Model file for the job. Use its own axes, mm. Face numbers are marked on the shaded views. A direction names the side the tool comes from. Give positions to 0.01 mm unless a question says otherwise; leave off trailing zeros. Write each loop counter-clockwise with the first axis right and the second up, starting at its lowest first coordinate (ties: lowest second). Pieces come first, ordered by that corner, then holes. Notation, with made-up numbers: M -18,85.5 L 34,85.5 A24 ccw 34,97.5 Z; hole C -27.75,71 d3. An arc over 180 degrees is marked long. Answer as a JSON object with one key per item and string values. Group by question number.
```python
from build123d import *

# Parameters (mm, degrees)
SKETCH1_R           = 7.9375
BOSS_EXTRUDE1_DEPTH = 1.524


with BuildPart() as part:
    # Sketch1 → Boss-Extrude1 (new body)
    with BuildSketch(Plane.XY):
        with Locations(Location((107.492585866, -0.762, 0), (0, 0, 180))):
            Circle(SKETCH1_R)
        Polygon((110.207675722, 0), (110.207675722, -1.524), (108.925853356, -1.524), (108.869130969, -1.622246056), (109.510042152, -2.732336789), (108.190219437, -3.494336789), (107.549308253, -2.384246056), (107.435863479, -2.384246056), (106.794952296, -3.494336789), (105.47512958, -2.732336789), (106.116040764, -1.622246056), (106.059318377, -1.524), (104.77749601, -1.524), (104.77749601, 0), (106.059318377, 0), (106.116040764, 0.098246056), (105.47512958, 1.208336789), (106.794952296, 1.970336789), (107.435863479, 0.860246056), (107.549308253, 0.860246056), (108.190219437, 1.970336789), (109.510042152, 1.208336789), (108.869130969, 0.098246056), (108.925853356, 0), align=None, mode=Mode.SUBTRACT)
    extrude(amount=BOSS_EXTRUDE1_DEPTH)


solid = part.part
```
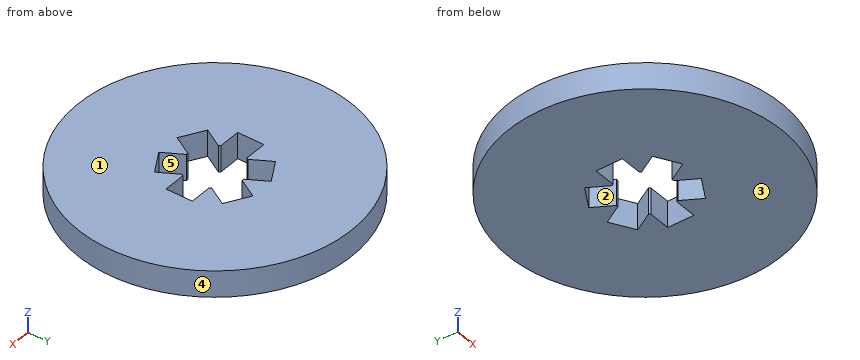
Q1. Slice it at B-B, the plane y = 3.25. Write the cut outline in (x, z), then the cut area to 3 significant figures.
Q2. Two-plate mould, pull along X, no slides. Class the marked faces 3, 4 and 5: +X half, -X half, draft (parallel to the pull), parting line (faces both ways), or undercut.
Q3. 3-axis set-ups, long thin cutter, end or side, ignore diameter. For the marked faces 1 and 2: which of +Z, -Z, +X, -X, +Y, -Y reach the whole face in a straight line?
Q4. Wall check: L1, parallel to Y at x = 107.5, z = 0.25; L2, parallel to X at y = -2.5, z = 0.6; L3, parallel to Y at x = 106, z = 1.15. Give the ranges that are in metal, low to high.
Q5. Drop flat-ended pins along their axis: P1, Ø1.5, axis at x = 111, y = -0.5, coming from the -Z side; P2, Ø0.6, axis at x = 109.5, z = 1, coming from the -Y side. Give the stop position or say it passes through.
Q6. Slice it at C-C, the plane x = 113.5. Write the cut outline in (y, z), then the cut area to 3 significant figures.
Solved:
{
 "1": {"outline": "M 100.64,0 L 114.34,0 L 114.34,1.52 L 100.64,1.52 Z", "area": "20.9 mm²"},
 "2": {"face 3": "draft", "face 4": "parting line", "face 5": "undercut"},
 "3": {"face 1": "+Z, +X, -X, +Y, -Y", "face 2": "+Z, -Z"},
 "4": {"L1": "y = -8.7 to -2.38, 0.86 to 7.18", "L2": "x = 99.75 to 105.61, 107.37 to 107.62, 109.38 to 115.24", "L3": "y = -8.56 to -3.04, -1.82 to -1.52, 0 to 0.3, 1.51 to 7.03"},
 "5": {"P1": "stops at z = 0", "P2": "stops at y = -8.51"},
 "6": {"outline": "M -5.95,0 L 4.43,0 L 4.43,1.52 L -5.95,1.52 Z", "area": "15.8 mm²"}
}
